Source: CAD feature listing. Evaluate the final solid. Frame: model axes, mm. Give positions to 0.01 mm unless a question says otherwise; leave off trailing zeros. Loops run counter-clockwise (first coordinate to the right, second up) from the corner with the lowest first, then second, coordinate; pieces in that order, holes last. Notation, with made-up numbers: M 55.5,18 L 65.5,18 A20 ccw 65.5,50 Z; hole C -4,79.25 d7. An arc over 180 degrees is marked long. Put each result on its own line as item: value. Start each with the question number.
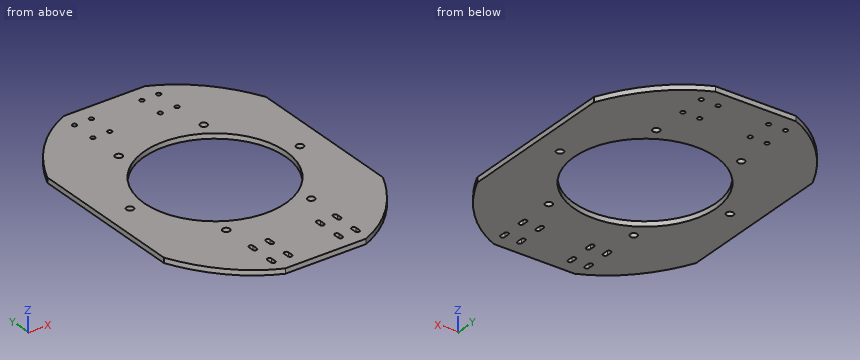
```python
from build123d import *

# Parameters (mm, degrees)
SKETCH_1_W          = 130
SKETCH_1_H          = 180
EXTRUDE_1_DEPTH     = 3
SKETCH_5_R          = 42
CUT_EXTRUDE_2_DEPTH = 10
SKETCH_8_R          = 2.1
CUT_EXTRUDE_5_DEPTH = 10
SKETCH_9_OUTSIDE_W  = 176.412
SKETCH_9_OUTSIDE_H  = 226.412
SKETCH_9_OUTSIDE_RX = 95
SKETCH_9_OUTSIDE_RY = 75
CUT_EXTRUDE_7_DEPTH = 10
CUT_EXTRUDE_8_REACH = 113.059
SKETCH_4_R          = 1.3


with BuildPart() as part:
    # 草图1 → 凸台-拉伸1 (new body)
    with BuildSketch(Plane.XY):
        Rectangle(SKETCH_1_W, SKETCH_1_H)
    extrude(amount=EXTRUDE_1_DEPTH)

    # 草图5 → 切除-拉伸2 (cut)
    with BuildSketch(Plane.XY.offset(3)):
        Circle(SKETCH_5_R)
    extrude(amount=-CUT_EXTRUDE_2_DEPTH, mode=Mode.SUBTRACT)

    # 草图8 → 切除-拉伸5 (cut)
    with BuildSketch(Plane.XY.offset(3)):
        with Locations((-50.45, 0)):
            Circle(SKETCH_8_R)
        with Locations((-25.225, 43.690981621)):
            Circle(SKETCH_8_R)
        with Locations((25.225, 43.690981621)):
            Circle(SKETCH_8_R)
        with Locations((50.45, 0)):
            Circle(SKETCH_8_R)
        with Locations((25.225, -43.690981621)):
            Circle(SKETCH_8_R)
        with Locations((-25.225, -43.690981621)):
            Circle(SKETCH_8_R)
    extrude(amount=-CUT_EXTRUDE_5_DEPTH, mode=Mode.SUBTRACT)

    # 草图9 outside → 切除-拉伸7 (cut)
    with BuildSketch(Plane.XY.offset(3)):
        Rectangle(SKETCH_9_OUTSIDE_W, SKETCH_9_OUTSIDE_H)
        with Locations(Location((0, 0), (0, 0, -90))):
            Ellipse(SKETCH_9_OUTSIDE_RX, SKETCH_9_OUTSIDE_RY, mode=Mode.SUBTRACT)
    extrude(amount=-CUT_EXTRUDE_7_DEPTH, mode=Mode.SUBTRACT)

    # 草图4 → 切除-拉伸8 (cut, up to next)
    with BuildSketch(Plane.XY.offset(3), mode=Mode.PRIVATE) as cut_extrude_8_sk1:
        with Locations((15, 65)):
            Circle(SKETCH_4_R)
    cut_extrude_8_tool1 = extrude(cut_extrude_8_sk1.sketch, amount=-CUT_EXTRUDE_8_REACH, mode=Mode.PRIVATE) & part.part
    # 草图4 → 切除-拉伸8 (cut, up to next)
    with BuildSketch(Plane.XY.offset(3), mode=Mode.PRIVATE) as cut_extrude_8_sk2:
        with Locations((25, 65)):
            Circle(SKETCH_4_R)
    cut_extrude_8_tool2 = extrude(cut_extrude_8_sk2.sketch, amount=-CUT_EXTRUDE_8_REACH, mode=Mode.PRIVATE) & part.part
    # 草图4 → 切除-拉伸8 (cut, up to next)
    with BuildSketch(Plane.XY.offset(3), mode=Mode.PRIVATE) as cut_extrude_8_sk3:
        with Locations((25, 80)):
            Circle(SKETCH_4_R)
    cut_extrude_8_tool3 = extrude(cut_extrude_8_sk3.sketch, amount=-CUT_EXTRUDE_8_REACH, mode=Mode.PRIVATE) & part.part
    # 草图4 → 切除-拉伸8 (cut, up to next)
    with BuildSketch(Plane.XY.offset(3), mode=Mode.PRIVATE) as cut_extrude_8_sk4:
        with Locations((15, 80)):
            Circle(SKETCH_4_R)
    cut_extrude_8_tool4 = extrude(cut_extrude_8_sk4.sketch, amount=-CUT_EXTRUDE_8_REACH, mode=Mode.PRIVATE) & part.part
    # 草图4 → 切除-拉伸8 (cut, up to next)
    with BuildSketch(Plane.XY.offset(3), mode=Mode.PRIVATE) as cut_extrude_8_sk5:
        with Locations((-25, 80)):
            Circle(SKETCH_4_R)
    cut_extrude_8_tool5 = extrude(cut_extrude_8_sk5.sketch, amount=-CUT_EXTRUDE_8_REACH, mode=Mode.PRIVATE) & part.part
    # 草图4 → 切除-拉伸8 (cut, up to next)
    with BuildSketch(Plane.XY.offset(3), mode=Mode.PRIVATE) as cut_extrude_8_sk6:
        with Locations((-15, 80)):
            Circle(SKETCH_4_R)
    cut_extrude_8_tool6 = extrude(cut_extrude_8_sk6.sketch, amount=-CUT_EXTRUDE_8_REACH, mode=Mode.PRIVATE) & part.part
    # 草图4 → 切除-拉伸8 (cut, up to next)
    with BuildSketch(Plane.XY.offset(3), mode=Mode.PRIVATE) as cut_extrude_8_sk7:
        with Locations((-15, 65)):
            Circle(SKETCH_4_R)
    cut_extrude_8_tool7 = extrude(cut_extrude_8_sk7.sketch, amount=-CUT_EXTRUDE_8_REACH, mode=Mode.PRIVATE) & part.part
    # 草图4 → 切除-拉伸8 (cut, up to next)
    with BuildSketch(Plane.XY.offset(3), mode=Mode.PRIVATE) as cut_extrude_8_sk8:
        with Locations((-25, 65)):
            Circle(SKETCH_4_R)
    cut_extrude_8_tool8 = extrude(cut_extrude_8_sk8.sketch, amount=-CUT_EXTRUDE_8_REACH, mode=Mode.PRIVATE) & part.part
    # 草图4 → 切除-拉伸8 (cut, up to next)
    with BuildSketch(Plane.XY.offset(3), mode=Mode.PRIVATE) as cut_extrude_8_sk9:
        with BuildLine():
            Line((-23.75, -63.5), (-23.75, -66.5))
            ThreePointArc((-23.75, -66.5), (-25, -67.75), (-26.25, -66.5))
            Line((-26.25, -66.5), (-26.25, -63.5))
            ThreePointArc((-26.25, -63.5), (-25, -62.25), (-23.75, -63.5))
        make_face()
    cut_extrude_8_tool9 = extrude(cut_extrude_8_sk9.sketch, amount=-CUT_EXTRUDE_8_REACH, mode=Mode.PRIVATE) & part.part
    # 草图4 → 切除-拉伸8 (cut, up to next)
    with BuildSketch(Plane.XY.offset(3), mode=Mode.PRIVATE) as cut_extrude_8_sk10:
        with BuildLine():
            Line((-13.75, -63.5), (-13.75, -66.5))
            ThreePointArc((-13.75, -66.5), (-15, -67.75), (-16.25, -66.5))
            Line((-16.25, -66.5), (-16.25, -63.5))
            ThreePointArc((-16.25, -63.5), (-15, -62.25), (-13.75, -63.5))
        make_face()
    cut_extrude_8_tool10 = extrude(cut_extrude_8_sk10.sketch, amount=-CUT_EXTRUDE_8_REACH, mode=Mode.PRIVATE) & part.part
    # 草图4 → 切除-拉伸8 (cut, up to next)
    with BuildSketch(Plane.XY.offset(3), mode=Mode.PRIVATE) as cut_extrude_8_sk11:
        with BuildLine():
            Line((-23.75, -78.5), (-23.75, -81.5))
            ThreePointArc((-23.75, -81.5), (-25, -82.75), (-26.25, -81.5))
            Line((-26.25, -81.5), (-26.25, -78.5))
            ThreePointArc((-26.25, -78.5), (-25, -77.25), (-23.75, -78.5))
        make_face()
    cut_extrude_8_tool11 = extrude(cut_extrude_8_sk11.sketch, amount=-CUT_EXTRUDE_8_REACH, mode=Mode.PRIVATE) & part.part
    # 草图4 → 切除-拉伸8 (cut, up to next)
    with BuildSketch(Plane.XY.offset(3), mode=Mode.PRIVATE) as cut_extrude_8_sk12:
        with BuildLine():
            Line((-13.75, -78.5), (-13.75, -81.5))
            ThreePointArc((-13.75, -81.5), (-15, -82.75), (-16.25, -81.5))
            Line((-16.25, -81.5), (-16.25, -78.5))
            ThreePointArc((-16.25, -78.5), (-15, -77.25), (-13.75, -78.5))
        make_face()
    cut_extrude_8_tool12 = extrude(cut_extrude_8_sk12.sketch, amount=-CUT_EXTRUDE_8_REACH, mode=Mode.PRIVATE) & part.part
    # 草图4 → 切除-拉伸8 (cut, up to next)
    with BuildSketch(Plane.XY.offset(3), mode=Mode.PRIVATE) as cut_extrude_8_sk13:
        with BuildLine():
            Line((13.75, -78.5), (13.75, -81.5))
            ThreePointArc((13.75, -81.5), (15, -82.75), (16.25, -81.5))
            Line((16.25, -81.5), (16.25, -78.5))
            ThreePointArc((16.25, -78.5), (15, -77.25), (13.75, -78.5))
        make_face()
    cut_extrude_8_tool13 = extrude(cut_extrude_8_sk13.sketch, amount=-CUT_EXTRUDE_8_REACH, mode=Mode.PRIVATE) & part.part
    # 草图4 → 切除-拉伸8 (cut, up to next)
    with BuildSketch(Plane.XY.offset(3), mode=Mode.PRIVATE) as cut_extrude_8_sk14:
        with BuildLine():
            Line((23.75, -78.5), (23.75, -81.5))
            ThreePointArc((23.75, -81.5), (25, -82.75), (26.25, -81.5))
            Line((26.25, -81.5), (26.25, -78.5))
            ThreePointArc((26.25, -78.5), (25, -77.25), (23.75, -78.5))
        make_face()
    cut_extrude_8_tool14 = extrude(cut_extrude_8_sk14.sketch, amount=-CUT_EXTRUDE_8_REACH, mode=Mode.PRIVATE) & part.part
    # 草图4 → 切除-拉伸8 (cut, up to next)
    with BuildSketch(Plane.XY.offset(3), mode=Mode.PRIVATE) as cut_extrude_8_sk15:
        with BuildLine():
            Line((23.75, -63.5), (23.75, -66.5))
            ThreePointArc((23.75, -66.5), (25, -67.75), (26.25, -66.5))
            Line((26.25, -66.5), (26.25, -63.5))
            ThreePointArc((26.25, -63.5), (25, -62.25), (23.75, -63.5))
        make_face()
    cut_extrude_8_tool15 = extrude(cut_extrude_8_sk15.sketch, amount=-CUT_EXTRUDE_8_REACH, mode=Mode.PRIVATE) & part.part
    # 草图4 → 切除-拉伸8 (cut, up to next)
    with BuildSketch(Plane.XY.offset(3), mode=Mode.PRIVATE) as cut_extrude_8_sk16:
        with BuildLine():
            Line((13.75, -63.5), (13.75, -66.5))
            ThreePointArc((13.75, -66.5), (15, -67.75), (16.25, -66.5))
            Line((16.25, -66.5), (16.25, -63.5))
            ThreePointArc((16.25, -63.5), (15, -62.25), (13.75, -63.5))
        make_face()
    cut_extrude_8_tool16 = extrude(cut_extrude_8_sk16.sketch, amount=-CUT_EXTRUDE_8_REACH, mode=Mode.PRIVATE) & part.part
    add(cut_extrude_8_tool1.solids().sort_by_distance((15, 65, 3))[0], mode=Mode.SUBTRACT)
    add(cut_extrude_8_tool2.solids().sort_by_distance((25, 65, 3))[0], mode=Mode.SUBTRACT)
    add(cut_extrude_8_tool3.solids().sort_by_distance((25, 80, 3))[0], mode=Mode.SUBTRACT)
    add(cut_extrude_8_tool4.solids().sort_by_distance((15, 80, 3))[0], mode=Mode.SUBTRACT)
    add(cut_extrude_8_tool5.solids().sort_by_distance((-25, 80, 3))[0], mode=Mode.SUBTRACT)
    add(cut_extrude_8_tool6.solids().sort_by_distance((-15, 80, 3))[0], mode=Mode.SUBTRACT)
    add(cut_extrude_8_tool7.solids().sort_by_distance((-15, 65, 3))[0], mode=Mode.SUBTRACT)
    add(cut_extrude_8_tool8.solids().sort_by_distance((-25, 65, 3))[0], mode=Mode.SUBTRACT)
    add(cut_extrude_8_tool9.solids().sort_by_distance((-25, -65, 3))[0], mode=Mode.SUBTRACT)
    add(cut_extrude_8_tool10.solids().sort_by_distance((-15, -65, 3))[0], mode=Mode.SUBTRACT)
    add(cut_extrude_8_tool11.solids().sort_by_distance((-25, -80, 3))[0], mode=Mode.SUBTRACT)
    add(cut_extrude_8_tool12.solids().sort_by_distance((-15, -80, 3))[0], mode=Mode.SUBTRACT)
    add(cut_extrude_8_tool13.solids().sort_by_distance((15, -80, 3))[0], mode=Mode.SUBTRACT)
    add(cut_extrude_8_tool14.solids().sort_by_distance((25, -80, 3))[0], mode=Mode.SUBTRACT)
    add(cut_extrude_8_tool15.solids().sort_by_distance((25, -65, 3))[0], mode=Mode.SUBTRACT)
    add(cut_extrude_8_tool16.solids().sort_by_distance((15, -65, 3))[0], mode=Mode.SUBTRACT)


solid = part.part
```
1. Section A-A, the plane x = 0. Output: boundary loops of the cut face in (y, z).
2. Contact query for flat-ended pins moving along their axis: pin 1 (0.9 mm diameter, centred on y = -80.5, z = 1.5, fed in from +X); pin 2 (1.5 mm diameter, centred on y = -80.5, z = 1.5, fed in from -X) (3 decimals). Output: stop coordinate, or through.
3. Section C-C, the plane x = -21. Output: boundary loops of the cut face in (y, z).
4. Section B-B, the plane z = 0.6. State how many separate pieces and enclosed holes the cut face has, plus the area to 3 significant figures.
5. Ray query, line 1 (X direction, y = 43.5, z = 2.05); line 2 (Y direction, x = 14.5, z = 2.3); line 3 (X direction, y = 65, z = 2.25). Return the intervals inside material, ascending.
Results found:
1. outline: M -90,0 L -42,0 L -42,3 L -90,3 Z; M 42,0 L 90,0 L 90,3 L 42,3 Z
2. pin 1: x = 40.39
2. pin 2: x = -40.755
3. outline: M -90,0 L -36.37,0 L -36.37,3 L -90,3 Z; M 36.37,0 L 90,0 L 90,3 L 36.37,3 Z
4. separate pieces: 1
4. enclosed holes: 23
4. area: 15,000 mm²
5. line 1: -65 to -27.32, -23.13 to 23.13, 27.32 to 65
5. line 2: -90 to -82.65, -77.35 to -67.65, -62.35 to -39.42, 39.42 to 63.8, 66.2 to 78.8, 81.2 to 90
5. line 3: -54.7 to -26.3, -23.7 to -16.3, -13.7 to 13.7, 16.3 to 23.7, 26.3 to 54.7
